For this review, use the dimensioned drawing (mm, ordinates from the lowest corner) and the shaded views. A direction names the side the tool comes from. Coordinates: 2 decimals unless noted, no trailing zeros.
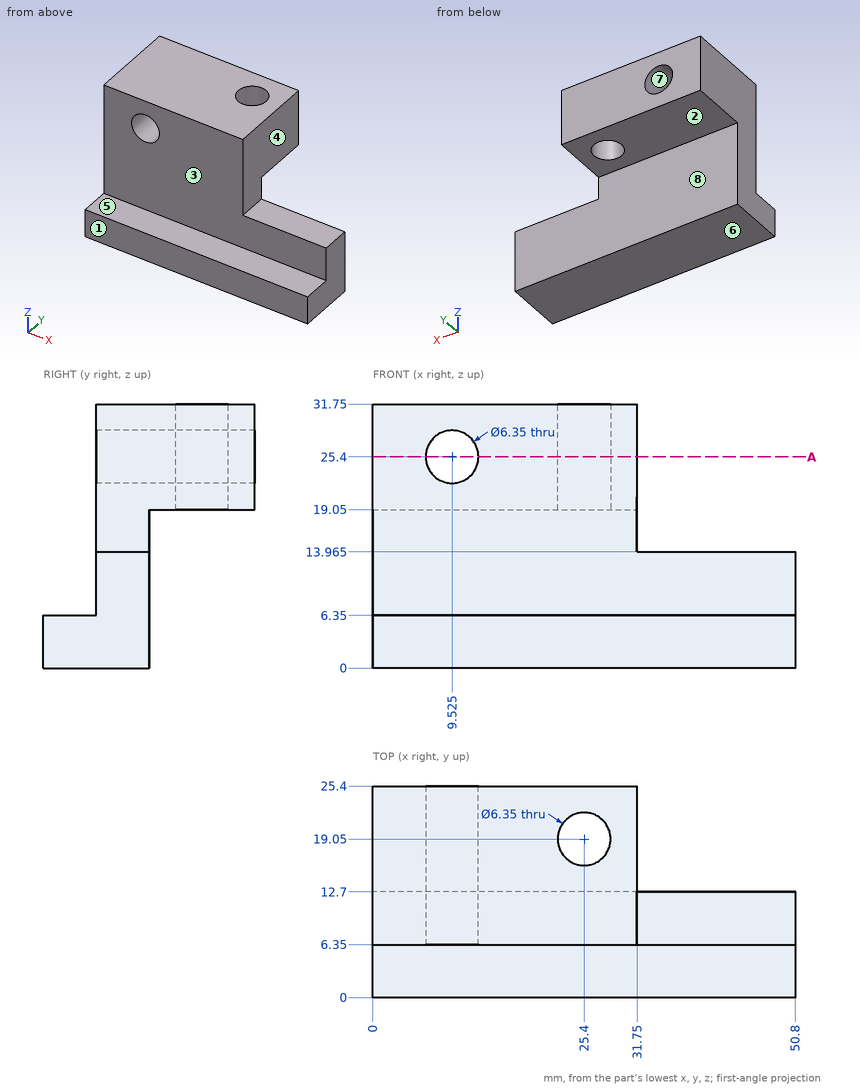
Item 1: Take a section at A-A, the plane z = 25.4. Count the separate pieces of the cut face and the enclosed holes in it, plus the area to 3 significant figures.
Solved:
separate pieces: 2
enclosed holes: 1
area: 452 mm2
Item 2: To check wall thickness, follow line 1 along X through (y, z) = (19.25, 30.5); line 2 along Y through (x, z) = (5.5, 10); line 3 along X through (y, z) = (10, 18). State the ranges of each line that lie inside material, in increasing order.
Solved:
line 1: x = 0 to 22.23, 28.57 to 31.75
line 2: y = 6.35 to 12.7
line 3: x = 0 to 31.75
Item 3: Mouldability with a two-part tool opening along Z and no side actions: class the marked faces 5, 6, 7 and 8 as pulls with the +Z half, pulls with the -Z half, needs draft (parallel to the pull), parting line crosses it, or undercut.
Solved:
face 5: pulls with the +Z half
face 6: pulls with the -Z half
face 7: undercut
face 8: needs draft
Item 4: For pin 1 (4 mm diameter, centred on x = 9.5, y = 16, fed in from -Z); pin 2 (9.5 mm diameter, centred on x = 37.5, z = 12, fed in from +Y); pin 3 (4 mm diameter, centred on x = 39.5, y = 3, fed in from +Z), all flat-tipped, find the tip position at first contact; note any pin that passes through.
Solved:
pin 1: stops at z = 19.05
pin 2: stops at y = 12.7
pin 3: stops at z = 6.35
Item 5: Machinability: for the marked faces 1, 2, 3 and 4, which of the approach directions +Z, -Z, +X, -X, +Y, -Y give a long, thin tool a straight path to every point of the face, cutting with its end or side? Answer none if there is none.
Solved:
face 1: +Z, -Z, +X, -X, -Y
face 2: -Z, +X, -X, +Y
face 3: +Z, +X, -X, -Y
face 4: +Z, +X, +Y, -Y
